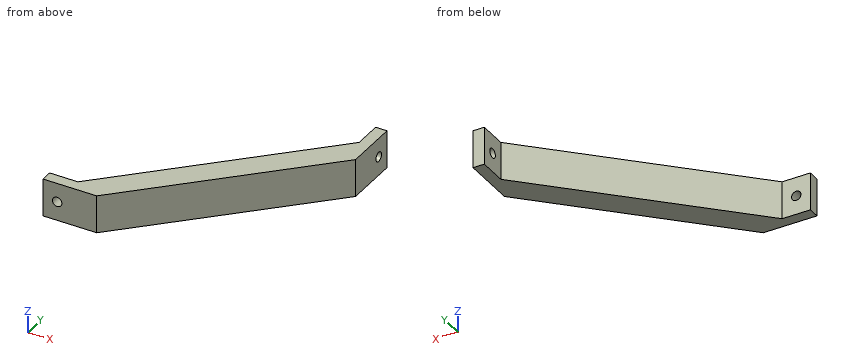
```python
from build123d import *

# Parameters (mm, degrees)
BOSS_EXTRUDE1_DEPTH = 20
SKETCH3_R           = 2.5
CUT_EXTRUDE1_DEPTH  = 20
SKETCH4_R           = 2.5
CUT_EXTRUDE2_DEPTH  = 20


with BuildPart() as part:
    # Sketch2 → Boss-Extrude1 (new body)
    with BuildSketch(Plane.XY):
        Polygon((-115, 0), (-115, 6), (-100, 6), (-6, 100), (-6, 115), (0, 115), (0, 86.541134144), (-86.541134144, 0), align=None)
    extrude(amount=BOSS_EXTRUDE1_DEPTH)

    # Sketch3 → Cut-Extrude1 (cut)
    with BuildSketch(Plane.ZY.offset(6)):
        with Locations((10, 107.5)):
            Circle(SKETCH3_R)
    extrude(amount=-CUT_EXTRUDE1_DEPTH, mode=Mode.SUBTRACT)

    # Sketch4 → Cut-Extrude2 (cut)
    with BuildSketch(Plane(origin=(0, 6, 0), x_dir=(1, 0, 0), z_dir=(0, 1, 0))):
        with Locations((-107.5, -10)):
            Circle(SKETCH4_R)
    extrude(amount=-CUT_EXTRUDE2_DEPTH, mode=Mode.SUBTRACT)


solid = part.part
```
Verification items for the finished model (mm, model axes). Coordinates: 2 decimals unless noted, no trailing zeros. Order: outer loops, then holes, each group sorted by start corner. A loop starts at its lowest first (then second) coordinate and runs counter-clockwise, first axis right, second up. Notation, with made-up numbers: (-24, -15.5) - (18, -15.5) arc R27 cw to (18, 13.5) - close; hole circle Ø4 at (28.5, 48.5). An arc over 180 degrees is marked (long way). Return JSON: item names as keys, results as strings.
(1) Thickness scan on line 1 along Z through (x, y) = (-107.5, 2.45); line 2 along Y through (x, z) = (-110, 6); line 3 along X through (y, z) = (1.75, 10). Record the ranges inside material, lowest first.
Filled sheet:
{"line 1": "z = 0 to 7.5, 12.5 to 20", "line 2": "y = 0 to 6", "line 3": "x = -115 to -110, -105 to -84.79"}
(2) Section check D-D, the plane y = 90.5. Record the cut outline in (x, z), and give its area (3 significant figures).
Filled sheet:
{"outline": "(-15.5, 0) - (0, 0) - (0, 20) - (-15.5, 20) - close", "area": "310 mm^2"}
(3) Section check B-B, the plane z = 10. Record the cut outline in (x, y), and give its area (3 significant figures).
Filled sheet:
{"outline": "(-115, 0) - (-110, 0) - (-110, 6) - (-115, 6) - close; (-105, 0) - (-86.54, 0) - (0, 86.54) - (0, 105) - (-6, 105) - (-6, 100) - (-100, 6) - (-105, 6) - close; (-6, 110) - (0, 110) - (0, 115) - (-6, 115) - close", "area": "1,960 mm^2"}
(4) Section check C-C, the plane y = 107.5. Record the cut outline in (x, z).
Filled sheet:
{"outline": "(-6, 0) - (0, 0) - (0, 7.5) - (-6, 7.5) - close; (-6, 12.5) - (0, 12.5) - (0, 20) - (-6, 20) - close"}
(5) Go/stop test with flat-tipped pins: pin 1 (4.5 mm diameter, centred on y = 110.5, z = 11.5, fed in from -X); pin 2 (10 mm diameter, centred on x = -32.5, z = 9.5, fed in from -Y); pin 3 (6 mm diameter, centred on x = -82.5, z = 14.5, fed in from -Y); pin 4 (4.5 mm diameter, centred on y = 107.5, z = 10, fed in from -X) (3 decimals). Record where each tip stops, or that it passes through.
Filled sheet:
{"pin 1": "stops at x = -6", "pin 2": "stops at y = 49.04", "pin 3": "stops at y = 1.04", "pin 4": "passes through"}
(6) Section check A-A, the plane x = -107.5. Record the cut outline in (y, z).
Filled sheet:
{"outline": "(0, 0) - (6, 0) - (6, 7.5) - (0, 7.5) - close; (0, 12.5) - (6, 12.5) - (6, 20) - (0, 20) - close"}
